Build history of the part. All positions in model axes, mm. Face numbers are marked on the shaded views. A direction names the side the tool comes from. Give positions to 0.01 mm unless a question says otherwise; leave off trailing zeros. Loops run counter-clockwise (first coordinate to the right, second up) from the corner with the lowest first, then second, coordinate; pieces in that order, holes last. Notation, with made-up numbers: M -27.75,52 L -12.75,52 A29 ccw -12.75,79 Z; hole C 42.5,23 d3. An arc over 180 degrees is marked long. Answer as a JSON object with one key per item and string values. Group by question number.
1. Mould opens along X. For the marked faces 3, 4 and 5 say: released by +X, released by -X, zero draft, split by the parting line, or undercut.
2. Slice it at D-D (x = 29). List the corners of the cut face in (y, z), then the cut area to 3 significant figures.
3. Drill centre lines: line 1 along X through (y, z) = (0.5, 23); line 2 along Y through (x, z) = (-12, -17); line 3 along X through (y, z) = (8.5, 20.5). Where is each one in solid material? Low to high. Write a range as [from, to].
4. Drop flat-ended pins along their axis: pin 1 Ø8 at (y, z) = (12.5, -28) entering from +X; pin 2 Ø4 at (y, z) = (13, -26.5) entering from -X; pin 3 Ø10 at (x, z) = (28, -18.5) entering from +Y. Give the stop position or say it passes through.
5. Slice it at A-A (z = 25.5). List the corners of the cut face in (x, y).
6. Slice it at C-C (z = -31.5). List the corners of the cut face in (x, y), then the cut area to 3 significant figures.
7. Slice it at B-B (x = -14.5). List the corners of the cut face in (y, z), then the cut area to 3 significant figures.
8. 3-axis set-ups, long thin cutter, end or side, ignore diameter. For the marked faces 1 and 2: which of +Z, -Z, +X, -X, +Y, -Y reach the whole face in a straight line?
Autodesk Fusion 360 part; units mm, degrees
sketch "Sketch1" plane through (0, 0, 0) normal (0, 1, 0) x (1, 0, 0)
  circle A0 centre (0, 0) radius 37.5
  line L0 (0, 37.5) -> (0, -37.5) construction
  line L1 (0, 0) -> (37.5, 0) construction
  circle A1 centre (0, 0) radius 26.5 construction
  line L2 (0, 0) -> (37.5, 0) construction
  line L3 (0, 0) -> (6.5118, -36.9303) construction
  line L4 (0, 0) -> (37.5, 0) construction
  line L5 (0, 0) -> (37.3573, -3.2683) construction
  line L6 (0, 0) -> (37.5, 0) construction
  line L7 (0, 0) -> (24.2558, -10.6728) construction
  line L8 (0, 0) -> (26.5, 0) construction
  line L9 (0, 0) -> (19.5378, -17.9031) construction
  line L10 (0, 0) -> (26.5, 0) construction
  line L11 (0, 0) -> (12.7462, -23.2333) construction
  line L12 (0, 0) -> (26.5, 0) construction
  circle A2 centre (26.3992, -2.3096) radius 2.5
  circle A3 centre (24.2558, -10.6728) radius 2.5
  circle A4 centre (19.5378, -17.9031) radius 2.5
  circle A5 centre (12.7462, -23.2333) radius 2.5
  circle A6 centre (4.6017, -26.0974) radius 2.5
  circle A7 centre (-4.6017, -26.0974) radius 2.5
  circle A8 centre (-12.7462, -23.2333) radius 2.5
  circle A9 centre (-19.5378, -17.9031) radius 2.5
  circle A10 centre (-24.2558, -10.6728) radius 2.5
  circle A11 centre (-26.3992, -2.3096) radius 2.5
  line L13 (0, 37.5) -> (0, 31.5)
  circle A12 centre (0, 31.5) radius 2.5
  circle A13 centre (-24.2558, -10.6728) radius 3.75
  circle A14 centre (24.2558, -10.6728) radius 3.75
  circle A15 centre (0, 31.5) radius 3.75
  circle A16 centre (-4.6017, -26.0974) radius 3.75
  circle A17 centre (4.6017, -26.0974) radius 3.75
  circle A18 centre (-12.7462, -23.2333) radius 3.75
  circle A19 centre (12.7462, -23.2333) radius 3.75
  circle A20 centre (-19.5378, -17.9031) radius 3.75
  circle A21 centre (-26.3992, -2.3096) radius 3.75
  circle A22 centre (26.3992, -2.3096) radius 3.75
  circle A23 centre (19.5378, -17.9031) radius 3.75
  circle A24 centre (0, 31.5) radius 6
  dimension "d1" = 75
  dimension "d5" = 80
  dimension "d6" = 5
  dimension "d9" = 23.75
  dimension "d10" = 42.5
  dimension "d11" = 61.25
  dimension "d12" = 5
  dimension "d13" = 5
  dimension "d14" = 5
  dimension "d15" = 5
  dimension "d16" = 5
  dimension "d29" = 6
  dimension "d39" = 7.5
  dimension "d40" = 7.5
  dimension "d41" = 7.5
  dimension "d44" = 7.5
  dimension "d45" = 7.5
  dimension "d46" = 7.5
  dimension "d47" = 7.5
  dimension "d52" = 7.5
  dimension "d53" = 7.5
  dimension "d58" = 7.5
  dimension "d63" = 7.5
  dimension "d66" = 12
extrude "Extrude1" add sketch "Sketch1" against normal blind 2.5 contours A12 | A15 | A24 | A0 | A2 | A3 | A4 | A5 | A6 | A7 | A8 | A9 | A10 | A11 | A13 | A14 | A16 | A17 | A18 | A19 | A20 | A21 | A22 | A23 makes body 1
extrude "Extrude11" add sketch "Sketch1" along normal blind 15 separate body contours A12 | A15 makes body 2
extrude "Extrude16" add sketch "Sketch1" along normal blind 15 contours A24 bodies 1 2
extrude "Extrude17" cut 1 faces at (0.6119, -2.5, 13.5914) along direction (0, 1, 0) blind 1 on bodies 1 bodies 1
extrude "Extrude21" add sketch "Sketch1" along normal blind 15 contours A5 | A8 | A18 | A19 bodies 1
sketch "Sketch4" plane through (0, 0, 0) normal (0, 0, 1) x (1, 0, 0)
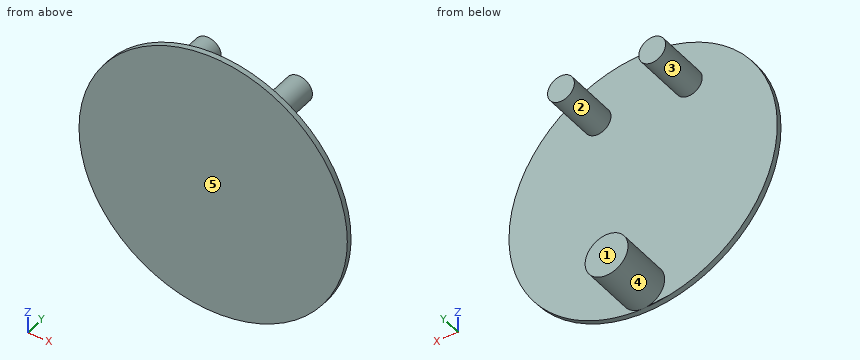
Established:
{
 "1": {"face 3": "undercut", "face 4": "split by the parting line", "face 5": "zero draft"},
 "2": {"outline": "M -1.5,-23.77 L 0,-23.77 L 0,23.77 L -1.5,23.77 Z", "area": "71.3 mm^2"},
 "3": {"line 1": "x = [-16.49, -9], [9, 16.49]", "line 2": "y = [-1.5, 0]", "line 3": "x = [-15.31, -10.18], [10.18, 15.31]"},
 "4": {"pin 1": "stops at x = 6", "pin 2": "stops at x = -5.2", "pin 3": "stops at y = 0"},
 "5": {"outline": "M -27.5,-1.5 L 27.5,-1.5 L 27.5,0 L 15.73,0 L 15.73,15 L 9.76,15 L 9.76,0 L -9.76,0 L -9.76,15 L -15.73,15 L -15.73,0 L -27.5,0 Z"},
 "6": {"outline": "M -20.35,-1.5 L 20.35,-1.5 L 20.35,0 L 6,0 L 6,15 L -6,15 L -6,0 L -20.35,0 Z", "area": "241 mm^2"},
 "7": {"outline": "M -1.5,-34.58 L 0,-34.58 L 0,19.92 L 15,19.92 L 15,26.55 L 0,26.55 L 0,34.58 L -1.5,34.58 Z", "area": "203 mm^2"},
 "8": {"face 1": "+Z, -Z, +X, -X, +Y", "face 2": "+Y"}
}
